from build123d import *

# Parameters (mm, degrees)
SKETCH1_R           = 1.5
BOSS_EXTRUDE1_DEPTH = 3.18
SKETCH2_R           = 1.5
CUT_EXTRUDE1_DEPTH  = 10
SKETCH3_R           = 5
CUT_EXTRUDE2_DEPTH  = 10
SKETCH4_W           = 20
SKETCH4_H           = 20
CUT_EXTRUDE3_DEPTH  = 10


with BuildPart() as part:
    # Sketch1 → Boss-Extrude1 (new body)
    with BuildSketch(Plane.XY):
        Polygon((-78.18, 75), (-12.5, 75), (-12.5, 78.18), (12.5, 78.18), (12.5, 75), (78.18, 75), (78.18, 12.5), (75, 12.5), (75, 1.5), (71, 1.5), (71, 4.5), (68, 4.5), (68, 1.5), (65.18, 1.5), (65.18, -1.5), (68, -1.5), (68, -4.5), (71, -4.5), (71, -1.5), (75, -1.5), (75, -12.5), (78.18, -12.5), (78.18, -75), (12.5, -75), (12.5, -78.18), (-12.5, -78.18), (-12.5, -75), (-78.18, -75), (-78.18, -12.5), (-75, -12.5), (-75, -1.5), (-71, -1.5), (-71, -4.5), (-68, -4.5), (-68, -1.5), (-65.18, -1.5), (-65.18, 1.5), (-68, 1.5), (-68, 4.5), (-71, 4.5), (-71, 1.5), (-75, 1.5), (-75, 12.5), (-78.18, 12.5), align=None)
        with Locations(Location((0, -76.59, 0), (0, 0, 180))):
            Circle(SKETCH1_R, mode=Mode.SUBTRACT)
        with Locations(Location((0, 76.59, 0), (0, 0, 180))):
            Circle(SKETCH1_R, mode=Mode.SUBTRACT)
    extrude(amount=BOSS_EXTRUDE1_DEPTH)

    # Sketch2 → Cut-Extrude1 (cut)
    with BuildSketch(Plane.XY.offset(3.18)):
        with Locations((32.5, 17.5)):
            Circle(SKETCH2_R)
        with Locations((32.5, -17.5)):
            Circle(SKETCH2_R)
        with Locations((-32.5, 17.5)):
            Circle(SKETCH2_R)
        with Locations((-32.5, -17.5)):
            Circle(SKETCH2_R)
    extrude(amount=-CUT_EXTRUDE1_DEPTH, mode=Mode.SUBTRACT)

    # Sketch3 → Cut-Extrude2 (cut)
    with BuildSketch(Plane.XY.offset(3.18)):
        Circle(SKETCH3_R)
    extrude(amount=-CUT_EXTRUDE2_DEPTH, mode=Mode.SUBTRACT)

    # Sketch4 → Cut-Extrude3 (cut)
    with BuildSketch(Plane.XY.offset(3.18)):
        with Locations((65, 0)):
            Rectangle(SKETCH4_W, SKETCH4_H)
    extrude(amount=-CUT_EXTRUDE3_DEPTH, mode=Mode.SUBTRACT)


solid = part.part
Check sheet for the modelled part. Datum: model origin and axes. Units: mm. Coordinates: 2 decimals unless noted, no trailing zeros. Write each loop counter-clockwise with the first axis right and the second up, starting at its lowest first coordinate (ties: lowest second). Pieces come first, ordered by that corner, then holes.
Item 1: Cross-section at B-B on x = 36. Record the boundary of the cut face in (y, z), then the cut area to 3 significant figures.
Numbers:
outline: (-75, 0) - (75, 0) - (75, 3.18) - (-75, 3.18) - close
area: 477 mm2
Item 2: Mould release check, pull along Y, two halves, no side actions. Record for faces 1 (the face through (-1.08, -4.88, 1.61)), 2 (the face through (18, 1, 0)): released by +Y, released by -Y, zero draft, split by the parting line, or undercut.
Numbers:
face 1: undercut
face 2: zero draft
Item 3: Depth check by flat-ended pin: pin 1 Ø1.5 at (x, z) = (-69.5, 2.5) entering from +Y; pin 2 Ø1.8 at (x, y) = (32.5, -17.5) entering from -Z; pin 3 Ø0.8 at (x, z) = (-67, 1.5) entering from -Y; pin 4 Ø0.9 at (y, z) = (3, 2) entering from +X. Enter the tip coordinate at first touch or a pass-through.
Numbers:
pin 1: stops at y = 75
pin 2: passes through
pin 3: stops at y = -75
pin 4: stops at x = 55
Item 4: Cross-section at A-A on z = 1.7. Count the separate pieces of the cut face and the enclosed holes in it, then the cut area to 3 significant figures.
Numbers:
separate pieces: 1
enclosed holes: 7
area: 22,900 mm2
Item 5: Scan lines: probe 1 along Y at (x, z) = (32.5, 2.55); probe 2 along Y at (x, z) = (68.5, 1.1); probe 3 along X at (y, z) = (76.59, 0.75). Record each from-to range of solid material in increasing order.
Numbers:
probe 1: y = -75 to -19, -16 to 16, 19 to 75
probe 2: y = -75 to -10, 10 to 75
probe 3: x = -12.5 to -1.5, 1.5 to 12.5
